```python
from build123d import *

# Parameters (mm, degrees)
SKETCH1_R           = 27.5
SKETCH1_R_2         = 4
BOSS_EXTRUDE1_DEPTH = 15
SKETCH1_3_R         = 27.5
SKETCH1_3_R_2       = 10
BOSS_EXTRUDE2_DEPTH = 34
SKETCH1_4_R         = 10
BOSS_EXTRUDE3_DEPTH = 124
BOSS_EXTRUDE4_START = 124
SKETCH1_5_R         = 5
BOSS_EXTRUDE4_DEPTH = 2


with BuildPart() as part:
    # Sketch1 → Boss-Extrude1 (new body)
    with BuildSketch(Plane.XY):
        with BuildLine():
            Line((-26, 31), (26, 31))
            ThreePointArc((26, 31), (29.535533906, 29.535533906), (31, 26))
            Line((31, 26), (31, -26))
            ThreePointArc((31, -26), (29.535533906, -29.535533906), (26, -31))
            Line((26, -31), (-26, -31))
            ThreePointArc((-26, -31), (-29.535533906, -29.535533906), (-31, -26))
            Line((-31, -26), (-31, 26))
            ThreePointArc((-31, 26), (-29.535533906, 29.535533906), (-26, 31))
        make_face()
        Circle(SKETCH1_R, mode=Mode.SUBTRACT)
        with Locations((-25.5, 25.5)):
            Circle(SKETCH1_R_2, mode=Mode.SUBTRACT)
        with Locations((25.5, 25.5)):
            Circle(SKETCH1_R_2, mode=Mode.SUBTRACT)
        with Locations((-25.5, -25.5)):
            Circle(SKETCH1_R_2, mode=Mode.SUBTRACT)
        with Locations((25.5, -25.5)):
            Circle(SKETCH1_R_2, mode=Mode.SUBTRACT)
    extrude(amount=BOSS_EXTRUDE1_DEPTH)

    # Sketch1<3> → Boss-Extrude2 (add)
    with BuildSketch(Plane.XY):
        Circle(SKETCH1_3_R)
        Circle(SKETCH1_3_R_2, mode=Mode.SUBTRACT)
    extrude(amount=BOSS_EXTRUDE2_DEPTH)

    # Sketch1<4> → Boss-Extrude3 (add)
    with BuildSketch(Plane.XY):
        Circle(SKETCH1_4_R)
    extrude(amount=BOSS_EXTRUDE3_DEPTH)

    # Sketch1<5> → Boss-Extrude4 (add)
    with BuildSketch(Plane.XY.offset(BOSS_EXTRUDE4_START)):
        Circle(SKETCH1_5_R)
    extrude(amount=BOSS_EXTRUDE4_DEPTH)


solid = part.part
```
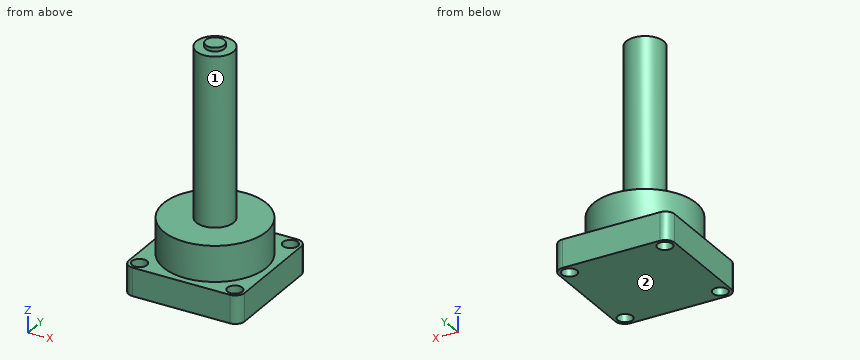
Verification items for the finished model (mm, model axes). Face numbers are marked on the shaded views. A direction names the side the tool comes from. Round coordinates to 2 decimals unless told otherwise and drop trailing zeros. Write each loop counter-clockwise with the first axis right and the second up, starting at its lowest first coordinate (ties: lowest second). Pieces come first, ordered by that corner, then holes. Notation, with made-up numbers: (86.5, -10.5) - (91.5, -10.5) arc R22 ccw to (91.5, 27.5) - close; hole circle Ø1 at (12.25, 51.25). An arc over 180 degrees is marked (long way). Answer as a JSON object with one key per item and string values. Group by question number.
Q1. Section check A-A, the plane x = 0. Enter the section's corners in (y, z), plus the area to 4 significant figures.
Q2. Section check C-C, the plane z = 32. Enter the section's corners in (x, y).
Q3. Go/stop test with flat-tipped pins: pin 1 Ø10.5 at (x, y) = (25.5, -25.5) entering from +Z; pin 2 Ø3 at (x, z) = (5, 82.5) entering from -Y; pin 3 Ø10 at (x, y) = (-15, 18.5) entering from +Z; pin 4 Ø2 at (y, z) = (-20.5, 35.5) entering from -X. Record where each tip stops, or that it passes through.
Q4. Section check D-D, the plane x = 17. Enter the section's corners in (y, z), plus the area to 3 significant figures.
Q5. Thickness scan on line 1 (Y direction, x = -25.5, z = 7); line 2 (X direction, y = -25, z = 7); line 3 (Z direction, x = 6.5, y = 22). Record the ranges inside material, lowest first.
Q6. Tool access check on the marked faces 1 and 2. Record the directions out of +Z, -Z, +X, -X, +Y, -Y that give a thin tool (end or side, any length) a straight path to the whole face; none if there is none.
Found:
{
 "1": {"outline": "(-31, 0) - (31, 0) - (31, 15) - (27.5, 15) - (27.5, 34) - (10, 34) - (10, 124) - (5, 124) - (5, 126) - (-5, 126) - (-5, 124) - (-10, 124) - (-10, 34) - (-27.5, 34) - (-27.5, 15) - (-31, 15) - close", "area": "3,795 mm^2"},
 "2": {"outline": "circle Ø55 at (0, 0)"},
 "3": {"pin 1": "stops at z = 15", "pin 2": "stops at y = -9.37", "pin 3": "stops at z = 34", "pin 4": "passes through"},
 "4": {"outline": "(-31, 0) - (31, 0) - (31, 15) - (21.62, 15) - (21.62, 34) - (-21.62, 34) - (-21.62, 15) - (-31, 15) - close", "area": "1,750 mm^2"},
 "5": {"line 1": "y = -31 to -29.5, -21.5 to 21.5, 29.5 to 31", "line 2": "x = -31 to -29.47, -21.53 to 21.53, 29.47 to 31", "line 3": "z = 0 to 34"},
 "6": {"face 1": "+Z", "face 2": "-Z, +X, -X, +Y, -Y"}
}
